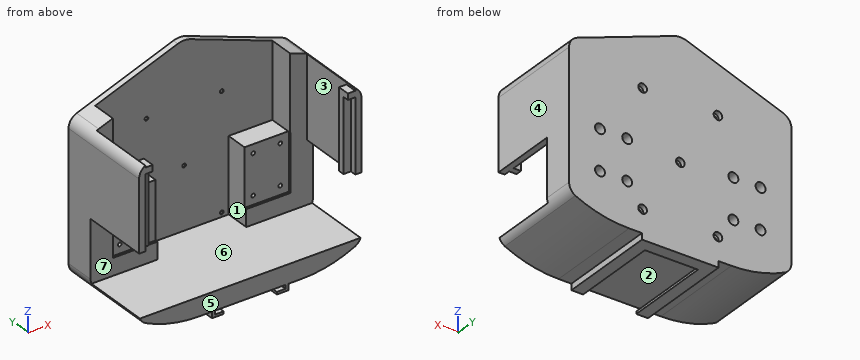
from build123d import *

# Parameters (mm, degrees)
BOSS_EXTRUDE1_DEPTH      = 40
BOSS_EXTRUDE1_DEPTH_BACK = 40
SKETCH1_W                = 180
SKETCH1_H                = 152.061
SHELL1_T                 = -5
SKETCH3_W                = 170
SKETCH3_H                = 142.061
BOSS_EXTRUDE2_DEPTH      = 20
SKETCH2_W                = 36
SKETCH2_H                = 55
CUT_EXTRUDE1_DEPTH       = 220
SKETCH4_W                = 36
SKETCH4_H                = 46.5
SKETCH4_R                = 1.5
CUT_EXTRUDE2_DEPTH       = 2
SKETCH4_3_R              = 1.5
CUT_EXTRUDE3_DEPTH       = 131.021678693
SKETCH5_W                = 159.952904784
SKETCH5_H                = 5
CUT_EXTRUDE4_DEPTH       = 63
SKETCH8_W                = 72
SKETCH8_H                = 29.937457508
CUT_EXTRUDE5_DEPTH       = 20
CUT_EXTRUDE7_DEPTH       = 102
SKETCH11_W               = 62
SKETCH11_H               = 5
BOSS_EXTRUDE3_DEPTH      = 80
SKETCH12_W               = 57
SKETCH12_H               = 3
SKETCH12_W_2             = 43
SKETCH12_H_2             = 2
CUT_EXTRUDE8_DEPTH       = 70
SKETCH13_W               = 57
SKETCH13_H               = 3
CUT_EXTRUDE9_DEPTH       = 7
SKETCH15_R               = 4
CUT_EXTRUDE10_DEPTH      = 17.5
SKETCH9_R                = 1.5
CUT_EXTRUDE11_DEPTH      = 10
BOSS_EXTRUDE4_DEPTH      = 10
SKETCH18_W               = 170
SKETCH18_H               = 5
SKETCH18_W_2             = 158
CUT_EXTRUDE12_DEPTH      = 114.303678916
FILLET3_R                = 100
FILLET2_R                = 10
FILLET1_R                = 15
SKETCH19_W               = 50
SKETCH19_H               = 65
CUT_EXTRUDE13_DEPTH      = 199
SKETCH20_W               = 6
SKETCH20_H               = 5
BOSS_EXTRUDE5_DEPTH      = 5
SKETCH24_R               = 3.5
CUT_EXTRUDE14_DEPTH      = 4


with BuildPart() as part:
    # Sketch1 → Boss-Extrude1 (new, two sides: drawn at the far end of the back side and taken through both)
    with BuildSketch(Plane(origin=(0, 0, 0), x_dir=(1, 0, 0), z_dir=(0, 1, 0)).offset(-BOSS_EXTRUDE1_DEPTH_BACK)):
        Rectangle(SKETCH1_W, SKETCH1_H)
    extrude(amount=BOSS_EXTRUDE1_DEPTH + BOSS_EXTRUDE1_DEPTH_BACK)

    # Shell1
    shell1_openings = [part.faces().sort_by_distance(p)[0] for p in [
        (0, -40, 0),
    ]]
    offset(amount=SHELL1_T, openings=shell1_openings, kind=Kind.INTERSECTION)

    # Sketch3 → Boss-Extrude2 (add)
    with BuildSketch(Plane.XZ.offset(-35)):
        Rectangle(SKETCH3_W, SKETCH3_H)
    extrude(amount=BOSS_EXTRUDE2_DEPTH)

    # Sketch2 → Cut-Extrude1 (cut)
    with BuildSketch(Plane.ZY.offset(90)):
        with Locations((-46.0305, -12.5)):
            Rectangle(SKETCH2_W, SKETCH2_H)
    extrude(amount=-CUT_EXTRUDE1_DEPTH, mode=Mode.SUBTRACT)

    # Sketch4 → Cut-Extrude2 (cut)
    with BuildSketch(Plane.XZ.offset(-15)):
        with Locations((-54, -34.0305)):
            Rectangle(SKETCH4_W, SKETCH4_H)
        with Locations(Location((-43, -50.2805, 0), (0, 0, 270))):
            Circle(SKETCH4_R, mode=Mode.SUBTRACT)
        with Locations(Location((-65, -50.2805, 0), (0, 0, 270))):
            Circle(SKETCH4_R, mode=Mode.SUBTRACT)
        with Locations(Location((-43, -17.7805, 0), (0, 0, 270))):
            Circle(SKETCH4_R, mode=Mode.SUBTRACT)
        with Locations(Location((-65, -17.7805, 0), (0, 0, 270))):
            Circle(SKETCH4_R, mode=Mode.SUBTRACT)
    cut_extrude2 = extrude(amount=-CUT_EXTRUDE2_DEPTH, mode=Mode.SUBTRACT)

    # Sketch4<3> → Cut-Extrude3 (cut, through all)
    with BuildSketch(Plane.XZ.offset(-15)):
        with BuildLine():
            Line((-65, -19.2805), (-65, -17.7805))
            Line((-65, -17.7805), (-63.5, -17.7805))
            ThreePointArc((-63.5, -17.7805), (-66.060660172, -16.719839828), (-65, -19.2805))
        make_face()
        with BuildLine():
            Line((-63.5, -17.7805), (-65, -17.7805))
            Line((-65, -17.7805), (-65, -19.2805))
            ThreePointArc((-65, -19.2805), (-63.939339828, -18.841160172), (-63.5, -17.7805))
        make_face()
        with BuildLine():
            Line((-65, -19.2805), (-65, -17.7805))
            Line((-65, -17.7805), (-63.5, -17.7805))
            ThreePointArc((-63.5, -17.7805), (-66.060660172, -16.719839828), (-65, -19.2805))
        make_face()
        with BuildLine():
            Line((-63.5, -17.7805), (-65, -17.7805))
            Line((-65, -17.7805), (-65, -19.2805))
            ThreePointArc((-65, -19.2805), (-63.939339828, -18.841160172), (-63.5, -17.7805))
        make_face()
        with Locations(Location((-43, -17.7805, 0), (0, 0, 270))):
            Circle(SKETCH4_3_R)
        with Locations(Location((-65, -50.2805, 0), (0, 0, 270))):
            Circle(SKETCH4_3_R)
        with Locations(Location((-43, -50.2805, 0), (0, 0, 270))):
            Circle(SKETCH4_3_R)
    cut_extrude3 = extrude(amount=-CUT_EXTRUDE3_DEPTH, mode=Mode.SUBTRACT)

    # Mirror2: Cut-Extrude2, Cut-Extrude3 across plane
    add(cut_extrude2.mirror(Plane(origin=(0, 0, 0), x_dir=(0, 0, 1), z_dir=(1, 0, 0))), mode=Mode.SUBTRACT)
    add(cut_extrude3.mirror(Plane(origin=(0, 0, 0), x_dir=(0, 0, 1), z_dir=(1, 0, 0))), mode=Mode.SUBTRACT)

    # Sketch5 → Cut-Extrude4 (cut)
    with BuildSketch(Plane.XZ.offset(-15)):
        with Locations((5.023547608, 73.5305)):
            Rectangle(SKETCH5_W, SKETCH5_H)
    extrude(amount=CUT_EXTRUDE4_DEPTH, mode=Mode.SUBTRACT)

    # Sketch8 → Cut-Extrude5 (cut)
    with BuildSketch(Plane.XZ.offset(-15)):
        Polygon((-36, -71.0305), (36, -71.0305), (36, -57.2805), (36, -10.7805), (-36, -10.7805), (-36, -57.2805), align=None)
        with Locations((0, 4.188228754)):
            Rectangle(SKETCH8_W, SKETCH8_H)
        Polygon((36, 19.156957508), (36, -10.7805), (71.419165144, -10.7805), (71.419165144, 76.0305), (-72, 76.0305), (-72, -10.7805), (-36, -10.7805), (-36, 19.156957508), align=None)
    extrude(amount=-CUT_EXTRUDE5_DEPTH, mode=Mode.SUBTRACT)

    # Sketch10 → Cut-Extrude7 (cut)
    with BuildSketch(Plane.XZ.offset(40)):
        Polygon((0, 76.0305), (90, 43.273178916), (90, 76.0305), align=None)
    cut_extrude7 = extrude(amount=-CUT_EXTRUDE7_DEPTH, mode=Mode.SUBTRACT)

    # Mirror3: Cut-Extrude7 across plane
    add(cut_extrude7.mirror(Plane(origin=(0, 0, 0), x_dir=(0, 0, 1), z_dir=(1, 0, 0))), mode=Mode.SUBTRACT)

    # Sketch11 → Boss-Extrude3 (add)
    with BuildSketch(Plane.XZ.offset(40)):
        Polygon((85, -86.0305), (85, -76.0305), (-85, -76.0305), (-85, -86.0305), (-31, -86.0305), (31, -86.0305), align=None)
        with Locations((0, -88.5305)):
            Rectangle(SKETCH11_W, SKETCH11_H)
    extrude(amount=-BOSS_EXTRUDE3_DEPTH)

    # Sketch12 → Cut-Extrude8 (cut)
    with BuildSketch(Plane.XZ.offset(40)):
        with Locations((0, -87.5305)):
            Rectangle(SKETCH12_W, SKETCH12_H)
        with Locations((0, -90.0305)):
            Rectangle(SKETCH12_W_2, SKETCH12_H_2)
    extrude(amount=-CUT_EXTRUDE8_DEPTH, mode=Mode.SUBTRACT)

    # Sketch13 → Cut-Extrude9 (cut)
    with BuildSketch(Plane.XZ.offset(-30)):
        with Locations((0, -87.5305)):
            Rectangle(SKETCH13_W, SKETCH13_H)
    extrude(amount=-CUT_EXTRUDE9_DEPTH, mode=Mode.SUBTRACT)

    # Sketch15 → Cut-Extrude10 (cut)
    with BuildSketch(Plane(origin=(0, 40, 0), x_dir=(1, 0, 0), z_dir=(0, 1, 0))):
        with Locations(Location((65, 17.7805, 0), (0, 0, 270))):
            Circle(SKETCH15_R)
        with Locations(Location((43, 17.7805, 0), (0, 0, 270))):
            Circle(SKETCH15_R)
        with Locations(Location((65, 50.2805, 0), (0, 0, 270))):
            Circle(SKETCH15_R)
        with Locations(Location((-43, 50.2805, 0), (0, 0, 90))):
            Circle(SKETCH15_R)
        with Locations(Location((43, 50.2805, 0), (0, 0, 270))):
            Circle(SKETCH15_R)
        with Locations(Location((-65, 50.2805, 0), (0, 0, 90))):
            Circle(SKETCH15_R)
        with Locations(Location((-43, 17.7805, 0), (0, 0, 90))):
            Circle(SKETCH15_R)
        with Locations(Location((-65, 17.7805, 0), (0, 0, 90))):
            Circle(SKETCH15_R)
    extrude(amount=-CUT_EXTRUDE10_DEPTH, mode=Mode.SUBTRACT)

    # Sketch9 → Cut-Extrude11 (cut)
    with BuildSketch(Plane.XZ.offset(-35)):
        with Locations(Location((30.5, -67.5305, 0), (0, 0, 270))):
            Circle(SKETCH9_R)
        with Locations(Location((-30.5, -67.5305, 0), (0, 0, 270))):
            Circle(SKETCH9_R)
        with Locations(Location((30.5, 25.4695, 0), (0, 0, 270))):
            Circle(SKETCH9_R)
        with Locations(Location((-30.5, 25.4695, 0), (0, 0, 270))):
            Circle(SKETCH9_R)
        with Locations(Location((0, -21.0305, 0), (0, 0, 270))):
            Circle(SKETCH9_R)
    extrude(amount=-CUT_EXTRUDE11_DEPTH, mode=Mode.SUBTRACT)

    # Sketch17 → Boss-Extrude4 (add)
    with BuildSketch(Plane.XZ.offset(30)):
        Polygon((90, 43.273178916), (-90, 43.273178916), (-90, -76.0305), (-85, -76.0305), (85, -76.0305), (90, -76.0305), align=None)
    extrude(amount=BOSS_EXTRUDE4_DEPTH)

    # Sketch18 → Cut-Extrude12 (cut)
    with BuildSketch(Plane.XY.offset(43.273178916)):
        with Locations((0, -37.5)):
            Rectangle(SKETCH18_W, SKETCH18_H)
        with Locations((0, -32.5)):
            Rectangle(SKETCH18_W_2, SKETCH18_H)
    extrude(amount=-CUT_EXTRUDE12_DEPTH, mode=Mode.SUBTRACT)

    # Fillet3
    # the kernel refuses this fillet: 100 mm, written as the material it takes off along each edge
    with BuildSketch(Plane(origin=(-85, -148.972473589, -86.0305), x_dir=(0, 0, 1), z_dir=(0, 1, 0))) as fillet3_piece_1:
        with BuildLine():
            CenterArc((100, 43.588989435), FILLET3_R, 180, 25.841932763)
            Line((0, 43.588989435), (0, 0))
            Line((0, 0), (10, 0))
        make_face()
    extrude(amount=297.944947177, mode=Mode.SUBTRACT)
    with BuildSketch(Plane(origin=(85, -148.972473589, -86.0305), x_dir=(-1, 0, 0), z_dir=(0, 1, 0))) as fillet3_piece_2:
        with BuildLine():
            CenterArc((43.588989435, 100), FILLET3_R, 244.158067237, 25.841932763)
            Line((0, 10), (0, 0))
            Line((0, 0), (43.588989435, 0))
        make_face()
    extrude(amount=297.944947177, mode=Mode.SUBTRACT)

    # Fillet2
    # the kernel refuses this fillet: 10 mm, written as the material it takes off along each edge
    with BuildSketch(Plane(origin=(90, -61.650635095, -76.0305), x_dir=(0, 0, 1), z_dir=(0, 1, 0)), Plane(origin=(-90, 61.650635095, -76.0305), x_dir=(0, 0, 1), z_dir=(0, -1, 0))) as fillet2_piece_1:
        with BuildLine():
            CenterArc((8.660254038, -10), FILLET2_R, 90, 60)
            Line((0, -5), (0, 0))
            Line((0, 0), (8.660254038, 0))
        make_face()
    extrude(amount=123.301270189, mode=Mode.SUBTRACT)
    with BuildSketch(Plane(origin=(-90, 57.505188455, 43.273178916), x_dir=(0.9396926207859103, 0, 0.34202014332566333), z_dir=(0, -1, 0)), Plane(origin=(90, -57.505188455, 43.273178916), x_dir=(-0.9396926207859106, 0, 0.34202014332566244), z_dir=(0, 1, 0))) as fillet2_piece_2:
        with BuildLine():
            CenterArc((FILLET2_R * 0.70020753821, -FILLET2_R), FILLET2_R, 90, 70)
            Line((-FILLET2_R * 0.239485082576, -FILLET2_R * 0.657979856674), (0, 0))
            Line((0, 0), (FILLET2_R * 0.70020753821, 0))
        make_face()
    extrude(amount=115.01037691, mode=Mode.SUBTRACT)

    # Fillet1
    fillet1_edges = [part.edges().sort_by_distance(p)[0] for p in [
        (0, 37.5, 76.0305),
    ]]
    fillet(fillet1_edges, radius=FILLET1_R)

    # Sketch19 → Cut-Extrude13 (cut)
    with BuildSketch(Plane(origin=(90, 0, 0), x_dir=(0, 0, -1), z_dir=(1, 0, 0))):
        with Locations((46.0305, -17.5)):
            Rectangle(SKETCH19_W, SKETCH19_H)
    extrude(amount=-CUT_EXTRUDE13_DEPTH, mode=Mode.SUBTRACT)

    # Sketch20 → Boss-Extrude5 (add)
    with BuildSketch(Plane.XZ.offset(35)):
        with Locations((-82, 40.773178916)):
            Rectangle(SKETCH20_W, SKETCH20_H)
        with Locations((82, 40.773178916)):
            Rectangle(SKETCH20_W, SKETCH20_H)
    extrude(amount=BOSS_EXTRUDE5_DEPTH)

    # Sketch24 → Cut-Extrude14 (cut)
    with BuildSketch(Plane(origin=(0, 40, 0), x_dir=(1, 0, 0), z_dir=(0, 1, 0))):
        with Locations(Location((0, 21.0305, 0), (0, 0, 270))):
            Circle(SKETCH24_R)
        with Locations(Location((-30.5, 67.5305, 0), (0, 0, 270))):
            Circle(SKETCH24_R)
        with Locations(Location((30.5, 67.5305, 0), (0, 0, 270))):
            Circle(SKETCH24_R)
        with Locations(Location((-30.5, -25.4695, 0), (0, 0, 270))):
            Circle(SKETCH24_R)
        with Locations(Location((30.5, -25.4695, 0), (0, 0, 270))):
            Circle(SKETCH24_R)
    extrude(amount=-CUT_EXTRUDE14_DEPTH, mode=Mode.SUBTRACT)


solid = part.part
Here's how the part is built. I have some questions about the finished solid (model axes, mm). Face numbers are marked on the shaded views. A direction names the side the tool comes from. Coordinates: 2 decimals unless noted, no trailing zeros. Order: outer loops, then holes, each group sorted by start corner. A loop starts at its lowest first (then second) coordinate and runs counter-clockwise, first axis right, second up. Notation, with made-up numbers: M 42,-18 L 69,-18 A35 cw 69,20 Z; hole C -35,-25.75 d3. An arc over 180 degrees is marked long. Answer as CSV lines item,"result". Start each with the question number.
1. On a 3-axis mill with a long thin cutter (end or side, diameter ignored), from which of +Z, -Z, +X, -X, +Y, -Y can I reach the whole of each face in a straight line? I mean the marked faces 1, 2, 3 and 4. Say none if no direction works.
2. I need wall thicknesses on line 1 (X direction, y = 28.5, z = -29.5); line 2 (X direction, y = -6, z = 23); line 3 (Z direction, x = 65, y = 18). Which ranges of each line are inside material? Lowest first, please. Write a range as [from, to].
3. I want a section at A-A, the plane y = -20.5. Write out the boundary of the cut face in (x, z).
4. For pin 1 (13 mm diameter, centred on x = 65, z = -17.78, fed in from -Y); pin 2 (2 mm diameter, centred on x = 22, y = 7.5, fed in from +Z); pin 3 (3.5 mm diameter, centred on x = 85.5, y = -25.5, fed in from -Z); pin 4 (12 mm diameter, centred on y = -30, z = 52, fed in from +X), each with a flat end and sliding along its axis, tell me the tip position at first contact or that it passes through.
5. We'd pull the mould along Y, two halves only. Please class the marked faces 5, 6 and 7: released by +Y, released by -Y, zero draft, split by the parting line, or undercut.
6. I want a section at C-C, the plane z = 53.5. Write out the boundary of the cut face in (x, y).
7. I want a section at B-B, the plane x = 51. Write out the boundary of the cut face in (y, z), and give its area (3 significant figures).
Recorded:
1,face 1,"+Z, -Y"
1,face 2,"-Y"
1,face 3,"+Z"
1,face 4,"+Z, -Z, +X, +Y, -Y"
2,line 1,"x = [-90, -36], [36, 90]"
2,line 2,"x = [-90, -85], [85, 90]"
2,line 3,"z = [-83.21, -51.78], [-48.78, -19.28], [-16.28, -10.78]"
3,outline,"M -90,-21.03 L -85,-21.03 L -85,44.93 A10 ccw -90,36.27 Z; M -89.31,-71.03 A10 ccw -85,-76.03 A100 ccw -41.41,-86.03 L -31,-86.03 L -31,-91.03 L -21.5,-91.03 L -21.5,-89.03 L -28.5,-89.03 L -28.5,-86.03 L 28.5,-86.03 L 28.5,-89.03 L 21.5,-89.03 L 21.5,-91.03 L 31,-91.03 L 31,-86.03 L 41.41,-86.03 A100 ccw 85,-76.03 A10 ccw 89.31,-71.03 Z; M 85,-21.03 L 90,-21.03 L 90,36.27 A10 ccw 85,44.93 Z"
4,pin 1,"stops at y = 17"
4,pin 2,"stops at z = -71.03"
4,pin 3,"stops at z = -76.63"
4,pin 4,"passes through"
5,face 5,"released by -Y"
5,face 6,"zero draft"
5,face 7,"undercut"
6,outline,"M -61.9,35 L 61.9,35 L 61.9,40 L -61.9,40 Z"
7,outline,"M -40,-85.57 L 40,-85.57 L 40,57.47 L 35,57.47 L 35,-10.78 L 17,-10.78 L 17,-57.28 L 15,-57.28 L 15,-71.03 L -40,-71.03 Z"
7,area,"2,920 mm2"
